Here's how the part is built. I have some questions about the finished solid (model axes, mm). Face numbers are marked on the shaded views. A direction names the side the tool comes from. Round coordinates to 2 decimals unless told otherwise and drop trailing zeros. Loops run counter-clockwise (first coordinate to the right, second up) from the corner with the lowest first, then second, coordinate; pieces in that order, holes last. Notation, with made-up numbers: M 46,49.5 L 55,49.5 A23 ccw 55,83.5 Z; hole C -12,65.5 d7. An arc over 180 degrees is marked long. Write each question's results on one line, items separated by ' | '. Start each with the question number.
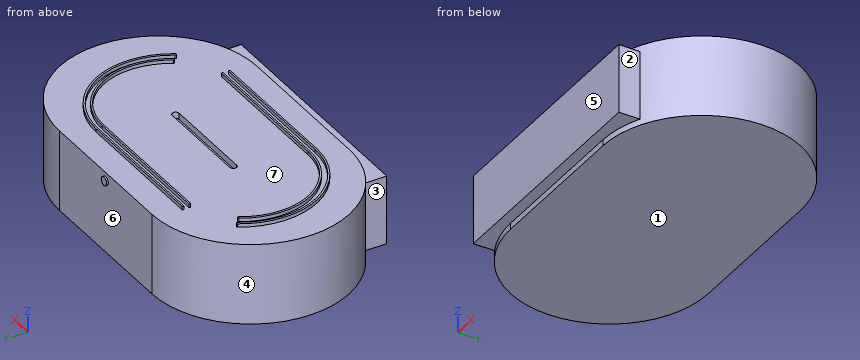
```python
from build123d import *

# Parameters (mm, degrees)
BOSS_EXTRUDE1_DEPTH = 119.38
SKETCH2_W           = 355.6
SKETCH2_H           = 101.6
BOSS_EXTRUDE2_DEPTH = 44.958
CUT_EXTRUDE1_DEPTH  = 9.652
SKETCH4_R           = 6.35
BOSS_EXTRUDE3_DEPTH = 2.54
BOSS_EXTRUDE4_DEPTH = 5.08


with BuildPart() as part:
    # Sketch1 → Boss-Extrude1 (new body)
    with BuildSketch(Plane.XY):
        with BuildLine():
            Line((-76.285439921, 56.800521538), (149.139560079, 56.800521538))
            ThreePointArc((149.139560079, 56.800521538), (294.427560079, -88.487478462), (149.139560079, -233.775478462))
            Line((149.139560079, -233.775478462), (-76.285439921, -233.775478462))
            ThreePointArc((-76.285439921, -233.775478462), (-221.573439921, -88.487478462), (-76.285439921, 56.800521538))
        make_face()
    extrude(amount=BOSS_EXTRUDE1_DEPTH)

    # Sketch2 → Boss-Extrude2 (add)
    with BuildSketch(Plane(origin=(0, -249.650478462, 0), x_dir=(-1, 0, 0), z_dir=(0, -1, 0))):
        with Locations((-36.427060079, -59.69)):
            Rectangle(SKETCH2_W, SKETCH2_H)
    extrude(amount=-BOSS_EXTRUDE2_DEPTH)

    # Sketch3 → Cut-Extrude1 (cut)
    with BuildSketch(Plane.XY.offset(119.38)):
        with BuildLine():
            Line((-33.895177701, -83.407478462), (106.749297859, -83.407478462))
            ThreePointArc((106.749297859, -83.407478462), (111.829297859, -88.487478462), (106.749297859, -93.567478462))
            Line((106.749297859, -93.567478462), (-33.895177701, -93.567478462))
            ThreePointArc((-33.895177701, -93.567478462), (-38.975177701, -88.487478462), (-33.895177701, -83.407478462))
        make_face()
    extrude(amount=-CUT_EXTRUDE1_DEPTH, mode=Mode.SUBTRACT)

    # Sketch4 → Boss-Extrude3 (add)
    with BuildSketch(Plane(origin=(0, 56.800521538, 0), x_dir=(1, 0, 0), z_dir=(0, 1, 0))):
        with Locations((36.427060079, -107.228428284)):
            Circle(SKETCH4_R)
    extrude(amount=BOSS_EXTRUDE3_DEPTH)

    # Sketch5 → Boss-Extrude4 (add)
    with BuildSketch(Plane.XY.offset(119.38)):
        with BuildLine():
            Line((-86.479093302, 18.700521538), (123.251136742, 18.700521538))
            ThreePointArc((123.251136742, 18.700521538), (223.504350955, -40.293834211), (220.612604828, -156.580887552))
            ThreePointArc((220.612604828, -156.580887552), (218.022957646, -157.022271916), (217.893868774, -154.398452419))
            ThreePointArc((217.893868774, -154.398452419), (220.780120028, -41.258888911), (123.251136742, 16.160521538))
            Line((123.251136742, 16.160521538), (-86.479093302, 16.160521538))
            ThreePointArc((-86.479093302, 16.160521538), (-87.749093302, 17.430521538), (-86.479093302, 18.700521538))
        make_face()
        with BuildLine():
            Line((-86.313359517, 8.540521538), (125.193739137, 8.540521538))
            ThreePointArc((125.193739137, 8.540521538), (215.020934696, -44.395432513), (212.23038132, -148.622843039))
            ThreePointArc((212.23038132, -148.622843039), (209.771349214, -149.194111608), (209.219629388, -146.730619796))
            ThreePointArc((209.219629388, -146.730619796), (212.668390329, -45.591104409), (125.608642701, 6.000521538))
            Line((125.608642701, 6.000521538), (-86.313359517, 6.000521538))
            ThreePointArc((-86.313359517, 6.000521538), (-87.583359517, 7.270521538), (-86.313359517, 8.540521538))
        make_face()
        with BuildLine():
            Line((150.962085254, -185.515478462), (-60.295843622, -185.515478462))
            ThreePointArc((-60.295843622, -185.515478462), (-150.123039181, -132.579524411), (-147.332485805, -28.352113885))
            ThreePointArc((-147.332485805, -28.352113885), (-144.876543413, -27.778907884), (-144.317816359, -30.238184654))
            ThreePointArc((-144.317816359, -30.238184654), (-147.45714929, -131.444373213), (-60.295843622, -182.975478462))
            Line((-60.295843622, -182.975478462), (150.962085254, -182.975478462))
            ThreePointArc((150.962085254, -182.975478462), (152.232085254, -184.245478462), (150.962085254, -185.515478462))
        make_face()
        with BuildLine():
            Line((150.962085254, -195.675478462), (-60.295843622, -195.675478462))
            ThreePointArc((-60.295843622, -195.675478462), (-160.549057836, -136.681122713), (-157.657311709, -20.394069372))
            ThreePointArc((-157.657311709, -20.394069372), (-155.067664526, -19.952685009), (-154.938575654, -22.576504505))
            ThreePointArc((-154.938575654, -22.576504505), (-157.824826909, -135.716068014), (-60.295843622, -193.135478462))
            Line((-60.295843622, -193.135478462), (150.962085254, -193.135478462))
            ThreePointArc((150.962085254, -193.135478462), (152.232085254, -194.405478462), (150.962085254, -195.675478462))
        make_face()
    extrude(amount=BOSS_EXTRUDE4_DEPTH)


solid = part.part
```
Item 1: If we section it at D-D on y = -109: Please give me the cut outline in (x, z).
Item 2: If we section it at A-A on x = 68.5: Please give me the cut outline in (y, z).
Item 3: If we section it at C-C on z = 75: Please give me the cut outline in (x, y), and give its area (3 significant figures).
Item 4: Which directions (+Z, -Z, +X, -X, +Y, -Y) give clear straight access to the entire face, cutting with the end or side of a thin tool? Please do the marked faces 1, 2 and 3.
Item 5: If we mould it in two halves opening along Y, with no side actions, what happens to the marked faces 4, 5, 6 and 7? For each: released by +Y, released by -Y, zero draft, split by the parting line, or undercut.
Item 6: I need wall thicknesses on L1, parallel to Y at x = 36.5, z = 38.5; L2, parallel to Z at x = 116, y = -202.5; L3, parallel to X at y = -90.5, z = 43.5. Which ranges of each line are inside material? Lowest first, please.
Item 7: I'm going to push flat-ended pins straight in: pin 1 (5 mm diameter, centred on x = 4.5, z = 113, fed in from +Y); pin 2 (2.5 mm diameter, centred on x = 21, z = 122, fed in from -Y); pin 3 (4.5 mm diameter, centred on x = 72, z = 4.5, fed in from -Y). Where does each tip first touch, or does it pass through?
Item 8: If we section it at B-B on y = -72.5: Please give me the cut outline in (x, z), and give its area (3 significant figures).
Numbers:
1) outline: M -220.12,0 L 292.97,0 L 292.97,119.38 L 237.19,119.38 L 237.19,124.46 L 233.95,124.46 L 233.95,119.38 L 226.8,119.38 L 226.8,124.46 L 223.6,124.46 L 223.6,119.38 L -156.45,119.38 L -156.45,124.46 L -159.59,124.46 L -159.59,119.38 L -168.42,119.38 L -168.42,124.46 L -171.5,124.46 L -171.5,119.38 L -220.12,119.38 Z
2) outline: M -249.65,8.89 L -233.78,8.89 L -233.78,0 L 56.8,0 L 56.8,119.38 L 18.7,119.38 L 18.7,124.46 L 16.16,124.46 L 16.16,119.38 L 8.54,119.38 L 8.54,124.46 L 6,124.46 L 6,119.38 L -83.41,119.38 L -83.41,109.73 L -93.57,109.73 L -93.57,119.38 L -182.98,119.38 L -182.98,124.46 L -185.52,124.46 L -185.52,119.38 L -193.14,119.38 L -193.14,124.46 L -195.68,124.46 L -195.68,119.38 L -233.78,119.38 L -233.78,110.49 L -249.65,110.49 Z
3) outline: M -141.37,-249.65 L 214.23,-249.65 L 214.23,-218.38 A145.29 ccw 149.14,56.8 L -76.29,56.8 A145.29 ccw -141.37,-218.38 Z | area: 138,000 mm²
4) face 1: -Z, +X, -X, +Y, -Y | face 2: +Z, -Z, +X, -Y | face 3: +Z, -Z, -X, -Y
5) face 4: split by the parting line | face 5: released by -Y | face 6: released by +Y | face 7: undercut
6) L1: -249.65 to 56.8 | L2: 0 to 119.38 | L3: -221.56 to 294.41
7) pin 1: y = 56.8 | pin 2: y = -195.68 | pin 3: y = -233.78
8) outline: M -220.69,0 L 293.55,0 L 293.55,119.38 L 235.5,119.38 L 235.5,124.46 L 232.42,124.46 L 232.42,119.38 L 225.57,119.38 L 225.57,124.46 L 222.67,124.46 L 222.67,119.38 L -159.17,119.38 L -159.17,124.46 L -162.46,124.46 L -162.46,119.38 L -171.46,119.38 L -171.46,124.46 L -174.66,124.46 L -174.66,119.38 L -220.69,119.38 Z | area: 61,500 mm²
